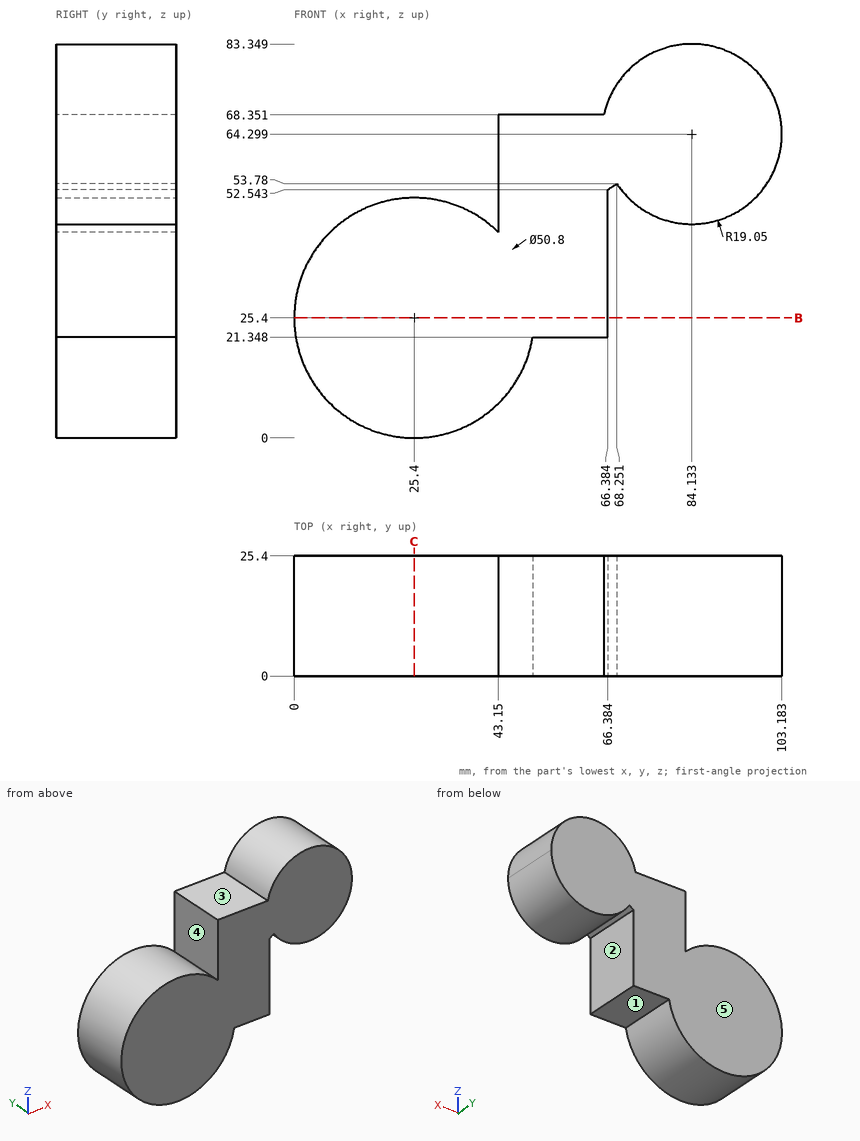
Geometry check sheet. Reference: drawing and pictorial views, mm from the part's lowest x, y, z. A direction names the side the tool comes from. Coordinates: 2 decimals unless noted, no trailing zeros. Order: outer loops, then holes, each group sorted by start corner. A loop starts at its lowest first (then second) coordinate and runs counter-clockwise, first axis right, second up.
Item 1: Section check C-C (x = 25.4). Enter the section's corners in (y, z).
Item 2: Mould release check, pull along X, two halves, no side actions. Record for the marked faces 4 and 5: released by +X, released by -X, zero draft, split by the parting line, or undercut.
Item 3: Scan lines: line 1 along Z through (x, y) = (65, 19.5); line 2 along Z through (x, y) = (27.5, 23.75); line 3 along X through (y, z) = (1.75, 21) (1 decimal). Record each from-to range of solid material in increasing order.
Item 4: Depth check by flat-ended pin: pin 1 (2 mm diameter, centred on y = 13.5, z = 18, fed in from +X); pin 2 (1.5 mm diameter, centred on x = 70.5, y = 9, fed in from -Z) (1 decimal); pin 3 (7.5 mm diameter, centred on y = 9, z = 36, fed in from +X). Enter the tip coordinate at first touch or a pass-through.
Item 5: Tool access check on the marked faces 1, 2 and 3. Record the directions out of +Z, -Z, +X, -X, +Y, -Y that give a thin tool (end or side, any length) a straight path to the whole face; none if there is none.
Item 6: Section check B-B (z = 25.4). Enter the section's corners in (x, y).
Check sheet entries:
1. outline: (0, 0) - (25.4, 0) - (25.4, 50.8) - (0, 50.8) - close
2. face 4: undercut
2. face 5: zero draft
3. line 1: z = 21.35 to 68.35
3. line 2: z = 0.09 to 50.71
3. line 3: x = 0.4 to 50.4
4. pin 1: stops at x = 49.98
4. pin 2: stops at z = 50.3
4. pin 3: stops at x = 66.38
5. face 1: -Z, +X, +Y, -Y
5. face 2: -Z, +Y, -Y
5. face 3: +Z, -X, +Y, -Y
6. outline: (0, 0) - (66.38, 0) - (66.38, 25.4) - (0, 25.4) - close
